Read the model definition and answer for the solid it produces. Units are mm, in the model's axes. A direction names the side the tool comes from. Give positions to 0.01 mm unless a question says otherwise; leave off trailing zeros. Order: outer loops, then holes, each group sorted by start corner. A loop starts at its lowest first (then second) coordinate and runs counter-clockwise, first axis right, second up. Notation, with made-up numbers: (-24.5, -1.75) -> (26.5, -1.75) arc R17 ccw to (26.5, 10.25) -> close; hole circle Ø9 at (1, 86). An arc over 180 degrees is marked (long way). One line per item, written item: value. Start each with the question number.
from build123d import *

# Parameters (mm, degrees)
F0_W     = 20
F0_H     = 8
F1_DEPTH = 16
F2_W     = 20
F2_H     = 2
F3_DEPTH = 8
F4_R     = 1.5
F5_DEPTH = 25


with BuildPart() as f1:
    # F0 (on Front) → F1 (new body)
    with BuildSketch(Plane.XZ):
        with Locations((-10, 4)):
            Rectangle(F0_W, F0_H)
    extrude(amount=F1_DEPTH)

    # F2 (on face) → F3 (cut)
    with BuildSketch(Plane.XZ.offset(16)):
        with Locations((-10, 4)):
            Rectangle(F2_W, F2_H)
    extrude(amount=-F3_DEPTH, mode=Mode.SUBTRACT)

    # F4 (on face) → F5 (cut)
    with BuildSketch(Plane.XY.offset(8)):
        with Locations((-16.5, -3.5)):
            Circle(F4_R)
        with Locations((-3.5, -3.5)):
            Circle(F4_R)
    extrude(amount=-F5_DEPTH, mode=Mode.SUBTRACT)


solid = f1.part
Item 1: Find section B-B on x = -16.5. Write down the section's boundary in (y, z).
Item 2: Find section A-A on y = -9. Write down the section's boundary in (x, z), then the cut area to 3 significant figures.
Item 3: A tool of negligible diameter and unlimited length cuts with its end or side. For faces 5 (the flat face through (-10, -12, 5)), 6 (the cylindrical face through (-18, -3.43, 4.06)), from which of +Z, -Z, +X, -X, +Y, -Y can it reach the whole face along a straight path? Write none if from no direction.
Item 4: Find the intervals of material crossed by line 1 (Z direction, x = -15.5, y = -10); line 2 (Y direction, x = -3.5, z = 4.5); line 3 (Y direction, x = -3.5, z = 5.75), in increasing order. Write a range as from..to.
Item 5: Find section D-D on y = -3.5. Write down the section's boundary in (x, z).
Item 6: Find section C-C on z = 6. Write down the section's boundary in (x, y).
Item 7: Flat-ended cylindrical pins translate along their axes: pin 1 (1 mm diameter, centred on x = -7, z = 4, fed in from -Y); pin 2 (8 mm diameter, centred on x = -4, y = -2.5, fed in from -Z). Find the tip coordinate at first contact, or state that the pin passes through.
Item 8: For a pull along Z with two mould halves and no side action, classify faces 1 (the flat face through (-10, -8, 0)), 2 (the flat face through (-20, -6, 4)), 3 (the flat face through (-10, -8, 8)), 4 (the flat face through (-10, -8, 4)) as +Z half, -Z half, draft (parallel to the pull), parting line (faces both ways), or undercut.
Checks:
1. outline: (-16, 0) -> (-5, 0) -> (-5, 8) -> (-16, 8) -> (-16, 5) -> (-8, 5) -> (-8, 3) -> (-16, 3) -> close; (-2, 0) -> (0, 0) -> (0, 8) -> (-2, 8) -> close
2. outline: (-20, 0) -> (0, 0) -> (0, 3) -> (-20, 3) -> close; (-20, 5) -> (0, 5) -> (0, 8) -> (-20, 8) -> close
2. area: 120 mm2
3. face 5: +X, -X, -Y
3. face 6: +Z, -Z
4. line 1: 0..3, 5..8
4. line 2: -8..-5, -2..0
4. line 3: -16..-5, -2..0
5. outline: (-20, 0) -> (-18, 0) -> (-18, 8) -> (-20, 8) -> close; (-15, 0) -> (-5, 0) -> (-5, 8) -> (-15, 8) -> close; (-2, 0) -> (0, 0) -> (0, 8) -> (-2, 8) -> close
6. outline: (-20, -16) -> (0, -16) -> (0, 0) -> (-20, 0) -> close; hole circle Ø3 at (-16.5, -3.5); hole circle Ø3 at (-3.5, -3.5)
7. pin 1: y = -8
7. pin 2: z = 0
8. face 1: -Z half
8. face 2: draft
8. face 3: +Z half
8. face 4: undercut
